CAD build for the part. Positions are in the model's coordinates, mm. Face numbers are marked on the shaded views. A direction names the side the tool comes from. Round coordinates to 2 decimals unless told otherwise and drop trailing zeros. Loops run counter-clockwise (first coordinate to the right, second up) from the corner with the lowest first, then second, coordinate; pieces in that order, holes last.
```python
from build123d import *

# Parameters (mm, degrees)
SKETCH1_W           = 51
SKETCH1_H           = 51
BOSS_EXTRUDE1_DEPTH = 14
SHELL1_T            = 1.2
CUT_EXTRUDE1_REACH  = 63.323
SKETCH3_W           = 8.833103678
SKETCH3_H           = 4.102185467
FILLET1_R           = 1
CHAMFER1_SIZE       = 1
FILLET2_R           = 1
BOSS_EXTRUDE2_DEPTH = 2.5
SKETCH4_3_R         = 1.09999934
BOSS_EXTRUDE3_DEPTH = 4.1
CUT_EXTRUDE3_REACH  = 63.323
SKETCH8_W           = 3
SKETCH8_H           = 1.5
FILLET3_R           = 1
SKETCH9_W           = 5
SKETCH9_H           = 1.5
CUT_EXTRUDE4_DEPTH  = 0.8
FILLET4_R           = 0.5
CUT_EXTRUDE5_REACH  = 63.323
SKETCH10_W          = 10
SKETCH10_H          = 7.000137798
SKETCH14_W          = 8.833103678
SKETCH14_H          = 0.4
CUT_EXTRUDE6_DEPTH  = 13


# Read off the part's stored shape, not the designer's step: Boss-Extrude2
with BuildPart() as part:
    # Sketch1 → Boss-Extrude1 (new body)
    with BuildSketch(Plane(origin=(0, 0, 0), x_dir=(1, 0, 0), z_dir=(0, 1, 0))):
        Rectangle(SKETCH1_W, SKETCH1_H)
    extrude(amount=BOSS_EXTRUDE1_DEPTH)

    # Shell1
    shell1_openings = [part.faces().sort_by_distance(p)[0] for p in [
        (0, 14, 0),
    ]]
    offset(amount=SHELL1_T, openings=shell1_openings, kind=Kind.INTERSECTION)

    # Sketch3 → Cut-Extrude1 (cut, up to next)
    with BuildSketch(Plane.XY.offset(26.7), mode=Mode.PRIVATE) as cut_extrude1_sk1:
        with Locations((-5.520237079, 4.278939715)):
            Rectangle(SKETCH3_W, SKETCH3_H)
    cut_extrude1_tool1 = extrude(cut_extrude1_sk1.sketch, amount=-CUT_EXTRUDE1_REACH, mode=Mode.PRIVATE) & part.part
    add(cut_extrude1_tool1.solids().sort_by_distance((-5.520237, 4.27894, 26.7))[0], mode=Mode.SUBTRACT)

    # Fillet1
    fillet1_edges = [part.edges().sort_by_distance(p)[0] for p in [
        (-1.10368524, 6.330032448, 26.1),
        (-9.936788918, 6.330032448, 26.1),
    ]]
    fillet(fillet1_edges, radius=FILLET1_R)

    # Chamfer1
    chamfer1_edges = [part.edges().sort_by_distance(p)[0] for p in [
        (-1.10368524, 2.227846981, 26.1),
        (-9.936788918, 2.227846981, 26.1),
    ]]
    chamfer(chamfer1_edges, length=CHAMFER1_SIZE)

    # Fillet2
    fillet2_edges = [part.edges().sort_by_distance(p)[0] for p in [
        (-1.10368524, 3.227846981, 26.1),
        (-8.936788918, 2.227846981, 26.1),
        (-2.10368524, 2.227846981, 26.1),
        (-9.936788918, 3.227846981, 26.1),
    ]]
    fillet(fillet2_edges, radius=FILLET2_R)

    # Boss-Extrude2 outline → Boss-Extrude2 (add)
    with BuildSketch(Plane(origin=(0, 0, 0), x_dir=(1, 0, 0), z_dir=(0, 1, 0))):
        with BuildLine():
            Line((25.5, 25.5), (22.50000961, 25.5))
            Line((22.50000961, 25.5), (22.50000961, 23.60000133))
            ThreePointArc((22.50000961, 23.60000133), (23.277821677, 23.277816289), (23.60000133, 22.50000199))
            Line((23.60000133, 22.50000199), (25.5, 22.50000199))
            Line((25.5, 22.50000199), (25.5, 25.5))
        make_face()
        with BuildLine():
            Line((-22.50000961, 23.60000133), (-22.50000961, 25.5))
            Line((-22.50000961, 25.5), (-25.5, 25.5))
            Line((-25.5, 25.5), (-25.5, 22.50000199))
            Line((-25.5, 22.50000199), (-23.60000895, 22.50000199))
            ThreePointArc((-23.60000895, 22.50000199), (-23.277826603, 23.277818983), (-22.50000961, 23.60000133))
        make_face()
        with BuildLine():
            Line((25.5, -25.5), (25.5, -22.50000199))
            Line((25.5, -22.50000199), (23.60000133, -22.50000199))
            ThreePointArc((23.60000133, -22.50000199), (23.277824371, -23.277821214), (22.50000961, -23.60000895))
            Line((22.50000961, -23.60000895), (22.50000961, -25.5))
            Line((22.50000961, -25.5), (25.5, -25.5))
        make_face()
        with BuildLine():
            Line((-23.60000895, -22.50000199), (-25.5, -22.50000199))
            Line((-25.5, -22.50000199), (-25.5, -25.5))
            Line((-25.5, -25.5), (-22.50000961, -25.5))
            Line((-22.50000961, -25.5), (-22.50000961, -23.60000895))
            ThreePointArc((-22.50000961, -23.60000895), (-23.277829297, -23.277823909), (-23.60000895, -22.50000199))
        make_face()
    extrude(amount=BOSS_EXTRUDE2_DEPTH)

    # Sketch4<3> → Boss-Extrude3 (add)
    with BuildSketch(Plane(origin=(0, 0, 0), x_dir=(1, 0, 0), z_dir=(0, 1, 0))):
        with Locations(Location((-22.50000961, 22.50000199, 0), (0, 0, 90))):
            Circle(SKETCH4_3_R)
        with Locations(Location((22.50000199, 22.50000199, 0), (0, 0, 89.999603096))):
            Circle(SKETCH4_3_R)
        with Locations(Location((22.50000199, -22.50000961, 0), (0, 0, 0.000396902))):
            Circle(SKETCH4_3_R)
        with Locations(Location((-22.50000961, -22.50000961, 0), (0, 0, 270))):
            Circle(SKETCH4_3_R)
    extrude(amount=BOSS_EXTRUDE3_DEPTH)

    # Sketch8 → Cut-Extrude3 (cut, up to next)
    with BuildSketch(Plane(origin=(26.7, 0, 0), x_dir=(0, 0, -1), z_dir=(1, 0, 0)), mode=Mode.PRIVATE) as cut_extrude3_sk1:
        with Locations((-20.2, 12.25)):
            Rectangle(SKETCH8_W, SKETCH8_H)
    cut_extrude3_tool1 = extrude(cut_extrude3_sk1.sketch, amount=-CUT_EXTRUDE3_REACH, mode=Mode.PRIVATE) & part.part
    # Sketch8 → Cut-Extrude3 (cut, up to next)
    with BuildSketch(Plane(origin=(26.7, 0, 0), x_dir=(0, 0, -1), z_dir=(1, 0, 0)), mode=Mode.PRIVATE) as cut_extrude3_sk2:
        with Locations((20.2, 12.25)):
            Rectangle(SKETCH8_W, SKETCH8_H)
    cut_extrude3_tool2 = extrude(cut_extrude3_sk2.sketch, amount=-CUT_EXTRUDE3_REACH, mode=Mode.PRIVATE) & part.part
    add(cut_extrude3_tool1.solids().sort_by_distance((26.7, 12.25, 20.2))[0], mode=Mode.SUBTRACT)
    add(cut_extrude3_tool2.solids().sort_by_distance((26.7, 12.25, -20.2))[0], mode=Mode.SUBTRACT)

    # Fillet3
    fillet3_edges = [part.edges().sort_by_distance(p)[0] for p in [
        (25.5, 13, 20.2),
        (25.5, 13, -20.2),
    ]]
    fillet(fillet3_edges, radius=FILLET3_R - 0.0001)  # a hair under: the kernel refuses the full size

    # Sketch9 → Cut-Extrude4 (cut)
    with BuildSketch(Plane(origin=(-25.5, 0, 0), x_dir=(0, 0, -1), z_dir=(1, 0, 0))):
        with Locations((0, 12.25)):
            Rectangle(SKETCH9_W, SKETCH9_H)
    extrude(amount=-CUT_EXTRUDE4_DEPTH, mode=Mode.SUBTRACT)

    # Fillet4
    fillet4_edges = [part.edges().sort_by_distance(p)[0] for p in [
        (-25.5, 13, 0),
    ]]
    fillet(fillet4_edges, radius=FILLET4_R)

    # Sketch10 → Cut-Extrude5 (cut, up to next)
    with BuildSketch(Plane(origin=(26.7, 0, 0), x_dir=(0, 0, -1), z_dir=(1, 0, 0)), mode=Mode.PRIVATE) as cut_extrude5_sk1:
        with Locations((1.575065653, 6.411548449)):
            Rectangle(SKETCH10_W, SKETCH10_H)
    cut_extrude5_tool1 = extrude(cut_extrude5_sk1.sketch, amount=-CUT_EXTRUDE5_REACH, mode=Mode.PRIVATE) & part.part
    add(cut_extrude5_tool1.solids().sort_by_distance((26.7, 6.411548, -1.575066))[0], mode=Mode.SUBTRACT)

    # Sketch14 → Cut-Extrude6 (cut)
    with BuildSketch(Plane(origin=(0, 14, 0), x_dir=(1, 0, 0), z_dir=(0, 1, 0))):
        with Locations((-5.520237079, -25.7)):
            Rectangle(SKETCH14_W, SKETCH14_H)
    extrude(amount=-CUT_EXTRUDE6_DEPTH, mode=Mode.SUBTRACT)


solid = part.part
```
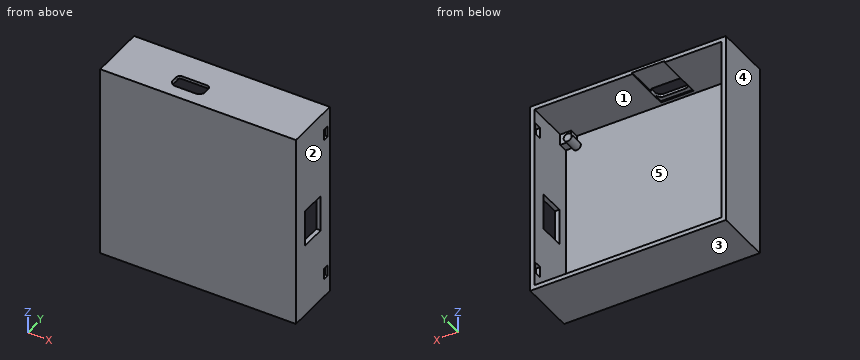
Item 1: Flat gauge pins, fed straight in: P1, Ø8, axis at x = 5.5, z = -2.5, coming from the +Y side; P2, Ø1.8, axis at x = 22.5, z = -22.5, coming from the +Y side. Where does each tip first touch, or does it go through?
Answers follow:
P1: stops at y = 0
P2: stops at y = 4.1
Item 2: Cut at A-A, the plane y = 9. Give the cut face in (x, z).
Answers follow:
outline: (-26.7, -26.7) - (26.7, -26.7) - (26.7, -6.58) - (25.5, -6.58) - (25.5, -25.5) - (-25.5, -25.5) - (-25.5, 25.5) - (-9.94, 25.5) - (-9.94, 25.9) - (-1.1, 25.9) - (-1.1, 25.5) - (25.5, 25.5) - (25.5, 3.42) - (26.7, 3.42) - (26.7, 26.7) - (-26.7, 26.7) - close
Item 3: 3-axis set-ups, long thin cutter, end or side, ignore diameter. For the marked faces 1 and 2: which of +Z, -Z, +X, -X, +Y, -Y reach the whole face in a straight line?
Answers follow:
face 1: +Y
face 2: +Z, -Z, +X, +Y, -Y
Item 4: Two-plate mould, pull along Z, no slides. Class the marked faces 3, 4 and 5: released by +Z, released by -Z, zero draft, split by the parting line, or undercut.
Answers follow:
face 3: released by -Z
face 4: zero draft
face 5: undercut
Item 5: Cut at B-B, the plane x = 1.5. Give the cut face in (y, z), plus the area to 3 significant figures.
Answers follow:
outline: (-1.2, -26.7) - (14, -26.7) - (14, -25.5) - (0, -25.5) - (0, 25.5) - (14, 25.5) - (14, 26.7) - (-1.2, 26.7) - close
area: 97.7 mm2
Item 6: Probe line 1 (Z direction, x = 9.5, y = 12.25); line 2 (Z direction, x = -2.5, y = 1.5). List the from-to ranges inside material, lowest first.
Answers follow:
line 1: z = -26.7 to -25.5, 25.5 to 26.7
line 2: z = -26.7 to -25.5, 25.9 to 26.7
Item 7: Cut at C-C, the plane z = -9. Give the cut face in (x, y), plus the area to 3 significant figures.
Answers follow:
outline: (-26.7, -1.2) - (26.7, -1.2) - (26.7, 14) - (25.5, 14) - (25.5, 0) - (-25.5, 0) - (-25.5, 14) - (-26.7, 14) - close
area: 97.7 mm2
